The model under review builds one solid part; all positions refer to its coordinate system, in mm. A direction names the side the tool comes from. Round coordinates to 2 decimals unless told otherwise and drop trailing zeros. Order: outer loops, then holes, each group sorted by start corner. A loop starts at its lowest first (then second) coordinate and runs counter-clockwise, first axis right, second up. Notation, with made-up numbers: (30.5, 55.25) -> (74.5, 55.25) arc R22 cw to (74.5, 74.25) -> close; hole circle Ø11 at (46, 43.5). An arc over 180 degrees is marked (long way). Return JSON: item names as keys, results as strings. Group by question number.
from build123d import *

# Parameters (mm, degrees)
SKETCH1_R                = 50.2
SKETCH1_R_2              = 40
BOSS_EXTRUDE1_DEPTH      = 12.7
CUT_EXTRUDE1_DEPTH       = 13.7
FILLET1_R                = 2
CIRPATTERN1_COUNT        = 4
FILLET1_OF_CIRPATTERN1_R = 2


with BuildPart() as part:
    # Sketch1 → Boss-Extrude1 (new body)
    with BuildSketch(Plane.XY):
        Circle(SKETCH1_R)
        Circle(SKETCH1_R_2, mode=Mode.SUBTRACT)
    extrude(amount=BOSS_EXTRUDE1_DEPTH)

    # Sketch2 → Cut-Extrude1 (cut, through all)
    with BuildSketch(Plane(origin=(0, 0, 0), x_dir=(-1, 0, 0), z_dir=(0, 0, -1))):
        with BuildLine():
            Line((-37.903382312, 22.639702058), (0, 0))
            Line((0, 0), (-22.639702058, 37.903382312))
            ThreePointArc((-22.639702058, 37.903382312), (-31.218764389, 31.218764389), (-37.903382312, 22.639702058))
        make_face()
        with BuildLine():
            Line((-46.112060645, 19.842325042), (-40.554730627, 17.450969136))
            ThreePointArc((-40.554730627, 17.450969136), (-44.15, 0), (-40.554730627, -17.450969136))
            Line((-40.554730627, -17.450969136), (-46.112060645, -19.842325042))
            ThreePointArc((-46.112060645, -19.842325042), (-50.2, 0), (-46.112060645, 19.842325042))
        make_face()
    cut_extrude1 = extrude(amount=-CUT_EXTRUDE1_DEPTH, mode=Mode.SUBTRACT)

    # Fillet1
    fillet1_edges = [part.edges().sort_by_distance(p)[0] for p in [
        (34.340550226, 20.511621344, 6.35),
        (20.511621344, 34.340550226, 6.35),
        (22.639702058, 37.903382312, 6.35),
        (37.903382312, 22.639702058, 6.35),
        (40.554730627, 17.450969136, 6.35),
        (40.554730627, -17.450969136, 6.35),
        (46.112060645, -19.842325042, 6.35),
        (46.112060645, 19.842325042, 6.35),
    ]]
    fillet(fillet1_edges, radius=FILLET1_R)

    # CirPattern1: Cut-Extrude1 ×4 about axis
    cirpattern1_axis = Axis((0, 0, 0), (0, 0, 1))
    for i in range(1, CIRPATTERN1_COUNT):
        add(cut_extrude1.rotate(cirpattern1_axis, i * 360 / CIRPATTERN1_COUNT), mode=Mode.SUBTRACT)

    # Fillet1 of CirPattern1
    fillet1_of_cirpattern1_edges = [part.edges().sort_by_distance(p)[0] for p in [
        (-20.511621344, 34.340550226, 6.35),
        (-34.340550226, 20.511621344, 6.35),
        (-37.903382312, 22.639702058, 6.35),
        (-22.639702058, 37.903382312, 6.35),
        (-17.450969136, 40.554730627, 6.35),
        (17.450969136, 40.554730627, 6.35),
        (19.842325042, 46.112060645, 6.35),
        (-19.842325042, 46.112060645, 6.35),
        (-34.340550226, -20.511621344, 6.35),
        (-20.511621344, -34.340550226, 6.35),
        (-22.639702058, -37.903382312, 6.35),
        (-37.903382312, -22.639702058, 6.35),
        (-40.554730627, -17.450969136, 6.35),
        (-40.554730627, 17.450969136, 6.35),
        (-46.112060645, 19.842325042, 6.35),
        (-46.112060645, -19.842325042, 6.35),
        (20.511621344, -34.340550226, 6.35),
        (34.340550226, -20.511621344, 6.35),
        (37.903382312, -22.639702058, 6.35),
        (22.639702058, -37.903382312, 6.35),
        (17.450969136, -40.554730627, 6.35),
        (-17.450969136, -40.554730627, 6.35),
        (-19.842325042, -46.112060645, 6.35),
        (19.842325042, -46.112060645, 6.35),
    ]]
    fillet(fillet1_of_cirpattern1_edges, radius=FILLET1_OF_CIRPATTERN1_R)


solid = part.part
Item 1: Consider section A-A on x = 7.5. State the section outline as (y, z) points, plus the area to 3 significant figures.
Item 2: Wall thickness on line 1 along Y through (x, z) = (1, 6.5); line 2 along Y through (x, z) = (-36.5, 7.25); line 3 along Y through (x, z) = (-29, 6): over which ranges is each line inside the solid? List them lowest first.
Item 3: For faces 1 (the face through (45.327, 20.192, 6.439)), 2 (the face through (-22.886, -37.075, 6.439)), list the 3-axis set-ups (+Z, -Z, +X, -X, +Y, -Y) from which the entire face can be reached by the end or side of a thin tool; tool diameter is ignored.
Item 4: Consider section B-B on y = -33. State the section outline as (x, z) points, plus the area to 3 significant figures.
Item 5: Insertion check: pin 1 Ø1 at (x, z) = (-13.5, 4.5) entering from -Y; pin 2 Ø1 at (y, z) = (-31.5, 6.5) entering from -X; pin 3 Ø1 at (x, z) = (16.5, 4) entering from +Y. Each pin has a flat end and moves straight along its axis. Give the tip position at first contact, or say it passes through.
Item 6: The part is to be moulded in two halves that separate along X. For faces 3 (the face through (-35.11, -20.31, 6.26)), 4 (the face through (20.192, -45.327, 6.439)), 5 (the face through (-41.31, -17.19, 6.44)), 6 (the face through (45.327, -20.192, 6.439)), say which applies: +X half, -X half, draft (parallel to the pull), parting line (faces both ways), or undercut.
Values:
{
 "1": {"outline": "(-43.51, 0) -> (-39.29, 0) -> (-39.29, 12.7) -> (-43.51, 12.7) -> close; (39.29, 0) -> (43.51, 0) -> (43.51, 12.7) -> (39.29, 12.7) -> close", "area": "107 mm^2"},
 "2": {"line 1": "-44.14 to -39.99, 39.99 to 44.14", "line 2": "-34.46 to -24.84, -21.86 to -16.36, 16.36 to 21.86, 24.84 to 34.46", "line 3": "-40.98 to -33.29, 33.29 to 40.98"},
 "3": {"face 1": "+Z, -Z, +X", "face 2": "+Z, -Z"},
 "4": {"outline": "(-37.83, 0) -> (-29.33, 0) -> (-29.33, 12.7) -> (-37.83, 12.7) -> close; (29.33, 0) -> (37.83, 0) -> (37.83, 12.7) -> (29.33, 12.7) -> close", "area": "216 mm^2"},
 "5": {"pin 1": "y = -42.19", "pin 2": "x = -39.48", "pin 3": "y = 41.24"},
 "6": {"face 3": "undercut", "face 4": "undercut", "face 5": "-X half", "face 6": "+X half"}
}
